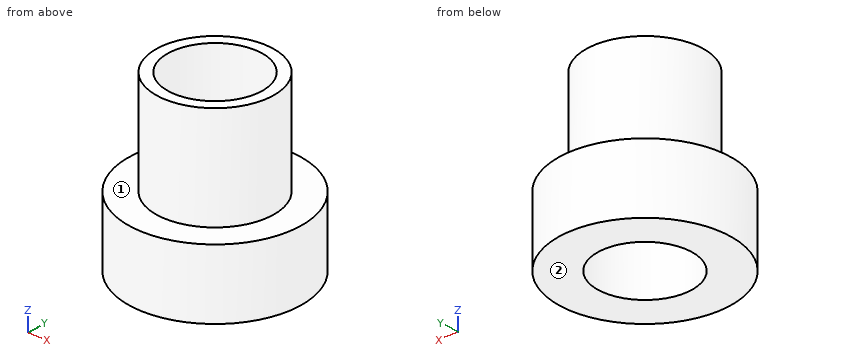
from build123d import *

# Parameters (mm, degrees)
SKETCH1_R           = 12.5
BOSS_EXTRUDE1_DEPTH = 12.5
SKETCH2_R           = 6.85
CUT_EXTRUDE1_DEPTH  = 25
SKETCH3_OUTSIDE_W   = 35.66
SKETCH3_OUTSIDE_H   = 35.66
SKETCH3_OUTSIDE_R   = 8.5
CUT_EXTRUDE2_DEPTH  = 15


with BuildPart() as part:
    # Sketch1 → Boss-Extrude1 (new, symmetric)
    with BuildSketch(Plane.XY):
        Circle(SKETCH1_R)
    extrude(amount=BOSS_EXTRUDE1_DEPTH, both=True)

    # Sketch2 → Cut-Extrude1 (cut)
    with BuildSketch(Plane(origin=(0, 0, -12.5), x_dir=(-1, 0, 0), z_dir=(0, 0, -1))):
        Circle(SKETCH2_R)
    extrude(amount=-CUT_EXTRUDE1_DEPTH, mode=Mode.SUBTRACT)

    # Sketch3 outside → Cut-Extrude2 (cut)
    with BuildSketch(Plane.XY.offset(12.5)):
        Rectangle(SKETCH3_OUTSIDE_W, SKETCH3_OUTSIDE_H)
        Circle(SKETCH3_OUTSIDE_R, mode=Mode.SUBTRACT)
    extrude(amount=-CUT_EXTRUDE2_DEPTH, mode=Mode.SUBTRACT)


solid = part.part
Could you check a few things on this model? Use its own coordinates, in mm. Face numbers are marked on the shaded views. A direction names the side the tool comes from. Round coordinates to 2 decimals unless told otherwise and drop trailing zeros. Order: outer loops, then holes, each group sorted by start corner. A loop starts at its lowest first (then second) coordinate and runs counter-clockwise, first axis right, second up. Notation, with made-up numbers: M 47.5,-7 L 84.5,-7 A15 cw 84.5,19 Z; hole C 71.25,10.5 d8. An arc over 180 degrees is marked long. One line per item, written item: value.
(1) I'm going to push flat-ended pins straight in: P1, Ø2, axis at y = -8.5, z = 0, coming from the -X side; P2, Ø10, axis at y = -7.5, z = -7, coming from the +X side; P3, Ø1.5, axis at x = -2.5, z = -1.5, coming from the +Y side; P4, Ø8, axis at x = 0, y = 0, coming from the +Z side. Where does each tip first touch, or does it pass through?
Ans:
P1: stops at x = -4
P2: stops at x = 12.25
P3: stops at y = 8.32
P4: passes through
(2) Imagine slicing it at D-D (y = 7.5). Write out the boundary of the cut face in (x, z).
Ans:
outline: M -10,-12.5 L 10,-12.5 L 10,-2.5 L 4,-2.5 L 4,12.5 L -4,12.5 L -4,-2.5 L -10,-2.5 Z
(3) Imagine slicing it at C-C (z = 3.5). Write out the boundary of the cut face in (x, y).
Ans:
outline: C 0,0 d17; hole C 0,0 d13.7
(4) I need wall thicknesses on line 1 along Y through (x, z) = (0, 6); line 2 along Y through (x, z) = (0, -5); line 3 along Z through (x, y) = (-1, 10.5). Which ranges of each line are inside material? Lowest first, please. Write a range as from..to.
Ans:
line 1: y = -8.5..-6.85, 6.85..8.5
line 2: y = -12.5..-6.85, 6.85..12.5
line 3: z = -12.5..-2.5
(5) Imagine slicing it at A-A (y = 0). Write out the boundary of the cut face in (x, z).
Ans:
outline: M -12.5,-12.5 L -6.85,-12.5 L -6.85,12.5 L -8.5,12.5 L -8.5,-2.5 L -12.5,-2.5 Z; M 6.85,-12.5 L 12.5,-12.5 L 12.5,-2.5 L 8.5,-2.5 L 8.5,12.5 L 6.85,12.5 Z
(6) Which directions (+Z, -Z, +X, -X, +Y, -Y) give clear straight access to the entire face, cutting with the end or side of a thin tool? Please do the marked faces 1 and 2.
Ans:
face 1: +Z
face 2: -Z, +X, -X, +Y, -Y
